from build123d import *

# Parameters (mm, degrees)
SKETCH1_W           = 25
SKETCH1_H           = 22
BOSS_EXTRUDE1_DEPTH = 60
CUT_EXTRUDE2_REACH  = 123.15
CUT_EXTRUDE3_REACH  = 123.15
SKETCH6_R           = 6.26
FILLET1_R           = 5
SKETCH2_R           = 2.5
BOSS_EXTRUDE2_DEPTH = 10
LPATTERN1_COUNT     = 6
LPATTERN1_PITCH     = 20
SKETCH3_R           = 2.5
BOSS_EXTRUDE3_DEPTH = 10
LPATTERN2_COUNT     = 6
LPATTERN2_PITCH     = 20
SKETCH4_R           = 7
CUT_EXTRUDE1_DEPTH  = 15


with BuildPart() as part:
    # Sketch1 → Boss-Extrude1 (new, symmetric)
    with BuildSketch(Plane(origin=(0, 0, 0), x_dir=(0, 0, -1), z_dir=(1, 0, 0))):
        Rectangle(SKETCH1_W, SKETCH1_H)
    extrude(amount=BOSS_EXTRUDE1_DEPTH, both=True)

    # Sketch5 → Cut-Extrude2 (cut, up to next)
    with BuildSketch(Plane(origin=(60, 0, 0), x_dir=(0, 0, -1), z_dir=(1, 0, 0)), mode=Mode.PRIVATE) as cut_extrude2_sk1:
        with BuildLine():
            Line((-13.743342576, 11), (-11.25, 11))
            Line((-11.25, 11), (-11.25, 6.005))
            ThreePointArc((-11.25, 6.005), (-23.092030441, 3.213639122), (-13.743342576, 11))
        make_face()
    cut_extrude2_tool1 = extrude(cut_extrude2_sk1.sketch, amount=-CUT_EXTRUDE2_REACH, mode=Mode.PRIVATE) & part.part
    add(cut_extrude2_tool1.solids().sort_by_distance((60, 6.117758, 17.335764))[0], mode=Mode.SUBTRACT)

    # Sketch6 → Cut-Extrude3 (cut, up to next)
    with BuildSketch(Plane.ZY.offset(60), mode=Mode.PRIVATE) as cut_extrude3_sk1:
        with Locations((17.5, -6.005)):
            Circle(SKETCH6_R)
    cut_extrude3_tool1 = extrude(cut_extrude3_sk1.sketch, amount=-CUT_EXTRUDE3_REACH, mode=Mode.PRIVATE) & part.part
    add(cut_extrude3_tool1.solids().sort_by_distance((-60, -6.005, 17.5))[0], mode=Mode.SUBTRACT)

    # Fillet1
    fillet1_edges = [part.edges().sort_by_distance(p)[0] for p in [
        (0, 11, 11.25),
    ]]
    fillet(fillet1_edges, radius=FILLET1_R)

    # Sketch2 → Boss-Extrude2 (add)
    with BuildSketch(Plane(origin=(60, 0, 0), x_dir=(0, 0, -1), z_dir=(1, 0, 0))):
        with BuildLine():
            Line((-17.250000617, 1.202041029), (-6.000000617, 1.202041029))
            Line((-6.000000617, 1.202041029), (-6.000000617, 11))
            Line((-6.000000617, 11), (-17.250000617, 11))
            ThreePointArc((-17.250000617, 11), (-21.250000617, 6.101020514), (-17.250000617, 1.202041029))
        make_face()
        with Locations((-16.250000617, 6.101020514)):
            Circle(SKETCH2_R, mode=Mode.SUBTRACT)
    boss_extrude2 = extrude(amount=-BOSS_EXTRUDE2_DEPTH)

    # LPattern1: Boss-Extrude2 ×6
    with Locations(*[(-i * LPATTERN1_PITCH, 0, 0) for i in range(1, LPATTERN1_COUNT)]):
        add(boss_extrude2)

    # Sketch3 → Boss-Extrude3 (add)
    with BuildSketch(Plane.ZY.offset(60)):
        with BuildLine():
            Line((17.24, -1.202041029), (12.5, -1.202041029))
            Line((12.5, -1.202041029), (12.5, -2.238356932))
            ThreePointArc((12.5, -2.238356932), (11.24, -6.005), (12.5, -9.771643068))
            Line((12.5, -9.771643068), (12.5, -11))
            Line((12.5, -11), (17.24, -11))
            ThreePointArc((17.24, -11), (21.24, -6.101020514), (17.24, -1.202041029))
        make_face()
        with Locations((16.24, -6.101020514)):
            Circle(SKETCH3_R, mode=Mode.SUBTRACT)
    boss_extrude3 = extrude(amount=-BOSS_EXTRUDE3_DEPTH)

    # LPattern2: Boss-Extrude3 ×6
    with Locations(*[(i * LPATTERN2_PITCH, 0, 0) for i in range(1, LPATTERN2_COUNT)]):
        add(boss_extrude3)

    # Sketch4 → Cut-Extrude1 (cut)
    with BuildSketch(Plane(origin=(0, 0, -12.5), x_dir=(-1, 0, 0), z_dir=(0, 0, -1))):
        with Locations(Location((0, 0, 0), (0, 0, 90))):
            Circle(SKETCH4_R)
    extrude(amount=-CUT_EXTRUDE1_DEPTH, mode=Mode.SUBTRACT)


solid = part.part
Read the model definition and answer for the solid it produces. Units are mm, in the model's axes. A direction names the side the tool comes from. Give positions to 0.01 mm unless a question says otherwise; leave off trailing zeros. Loops run counter-clockwise (first coordinate to the right, second up) from the corner with the lowest first, then second, coordinate; pieces in that order, holes last. Notation, with made-up numbers: (10, 76.25) -> (31, 76.25) arc R17 ccw to (31, 99.25) -> close; hole circle Ø9 at (-21, 52.5). An arc over 180 degrees is marked (long way). Use a Markdown table: item, result.
Q1. Section A-A, the plane y = 0 is taken. Determine the outline of the cut face in (x, z).
Solved:
| item | result |
|---|---|
| outline | (-60, -12.5) -> (-7, -12.5) -> (-7, 2.5) -> (7, 2.5) -> (7, -12.5) -> (60, -12.5) -> (60, 12.5) -> (-60, 12.5) -> close |
Q2. Section B-B, the plane z = -3.5 is taken. Determine the outline of the cut face in (x, y).
Solved:
| item | result |
|---|---|
| outline | (-60, -11) -> (60, -11) -> (60, 11) -> (-60, 11) -> close; hole circle Ø14 at (0, 0) |
Q3. Section C-C, the plane x = -47 is taken. Determine the outline of the cut face in (y, z) (3 decimals).
Solved:
| item | result |
|---|---|
| outline | (-11, -12.5) -> (11, -12.5) -> (11, 17.25) arc R5 ccw to (1.202, 17.25) -> (1.202, 12.5) -> (-2.238, 12.5) arc R6.26 cw to (-9.772, 12.5) -> (-11, 12.5) -> close; hole circle Ø5 at (6.101, 16.25) |
Q4. Determine the mould class of faces 1 (the face through (1, 11, -1)), 2 (the face through (35.07, 6.2, 21.25)), 3 (the face through (54.93, -5.95, 11.24)) for opening direction Y: pulls with the +Y half, pulls with the -Y half, needs draft (parallel to the pull), parting line crosses it, or undercut.
Solved:
| item | result |
|---|---|
| face 1 | pulls with the +Y half |
| face 2 | parting line crosses it |
| face 3 | undercut |
Q5. Find the intervals of material crossed by line 1 along Y through (x, z) = (5, 16.24); line 2 along Y through (x, z) = (34.5, 16.25); line 3 along Z through (x, y) = (-24.5, -0.5), in increasing order.
Solved:
| item | result |
|---|---|
| line 1 | y = -11 to -8.6, -3.6 to -1.2 |
| line 2 | y = 1.2 to 3.6, 8.6 to 11 |
| line 3 | z = -12.5 to 12.5 |
Q6. Each of these flat-tipped pins is pushed along its axis until it touches: pin 1 (5 mm diameter, centred on y = 7.5, z = 14, fed in from -X); pin 2 (1.4 mm diameter, centred on x = -12.5, z = 15.5, fed in from +Y); pin 3 (2.5 mm diameter, centred on x = 37, z = 14, fed in from -Y). Where does it stop, or does it pass through?
Solved:
| item | result |
|---|---|
| pin 1 | stops at x = -50 |
| pin 2 | stops at y = -1.2 |
| pin 3 | stops at y = 1.2 |
Q7. Section D-D, the plane y = -5 is taken. Count the separate pieces of the cut face and the enclosed holes in it, then the cut area to 3 significant figures.
Solved:
| item | result |
|---|---|
| separate pieces | 7 |
| enclosed holes | 0 |
| area | 3,030 mm^2 |
Q8. A tool of negligible diameter and unlimited length cuts with its end or side. For faces 4 (the face through (5, -1.202, 15)), 5 (the face through (0, 0, 2.5)), 6 (the face through (25.07, 4.054, 11.562)), 7 (the face through (-50, 7.26, 13.86)), from which of +Z, -Z, +X, -X, +Y, -Y can it reach the whole face along a straight path? Write none if from no direction.
Solved:
| item | result |
|---|---|
| face 4 | +Z, +X, -X, +Y |
| face 5 | -Z |
| face 6 | +Z, +Y |
| face 7 | +Z, -X, +Y |
